Can you work these out from the model? Positions are in its coordinate system, mm. A direction names the side the tool comes from. Give positions to 0.01 mm unless a question says otherwise; leave off trailing zeros. Write each loop counter-clockwise with the first axis right and the second up, starting at its lowest first coordinate (ties: lowest second). Pieces come first, ordered by that corner, then holes.
from build123d import *

# Parameters (mm, degrees)
F0_W     = 304.8
F0_H     = 6.35
F1_DEPTH = 50.8
F3_DEPTH = 0.8125
F5_DEPTH = 20.6502


# Not quite as in the source:
# - a pattern or mirror of a feature is missing from the dataset's text; its kind, count and spacing are read off the source's solid


with BuildPart() as f1:
    # F0 (on Right) → F1 (new body)
    with BuildSketch(Plane.YZ):
        with BuildLine():
            Line((-304.8, 6.35), (0, 6.35))
            Line((0, 6.35), (0, 19.05))
            ThreePointArc((0, 19.05), (-152.4, 44.45), (-304.8, 19.05))
            Line((-304.8, 19.05), (-304.8, 6.35))
        make_face()
        with BuildLine():
            ThreePointArc((-304.8, 19.05), (-152.4, 44.45), (0, 19.05))
            Line((0, 19.05), (0, 25.4))
            ThreePointArc((0, 25.4), (-152.4, 50.8), (-304.8, 25.4))
            Line((-304.8, 25.4), (-304.8, 19.05))
        make_face()
        with Locations((-152.4, 3.175)):
            Rectangle(F0_W, F0_H)
    extrude(amount=F1_DEPTH)

    # F2 (on face) → F3 (cut)
    with BuildSketch(Plane.YZ.offset(50.8)):
        with BuildLine():
            Line((0, 6.35), (0, 19.05))
            ThreePointArc((0, 19.05), (-152.4, 44.45), (-304.8, 19.05))
            Line((-304.8, 19.05), (-304.8, 6.35))
            Line((-304.8, 6.35), (0, 6.35))
        make_face()
    extrude(amount=-F3_DEPTH, mode=Mode.SUBTRACT)

    # F4 (on face) → F5 (cut)
    with BuildSketch(Plane(origin=(0, 0, 0), x_dir=(0, -1, 0), z_dir=(-1, 0, 0))):
        with BuildLine():
            Line((304.8, 6.35), (304.8, 19.05))
            ThreePointArc((304.8, 19.05), (152.4, 44.45), (0, 19.05))
            Line((0, 19.05), (0, 6.35))
            Line((0, 6.35), (304.8, 6.35))
        make_face()
    f5 = extrude(amount=-F5_DEPTH, mode=Mode.SUBTRACT)

    # F5_copies: F5 across plane
    add(f5.mirror(Plane(origin=(25.40635, 0, 0), x_dir=(0, 0, 1), z_dir=(1, 0, 0))), mode=Mode.SUBTRACT)


solid = f1.part
(1) Imagine slicing it at B-B, the plane y = -109. Write out the boundary of the cut face in (x, z), plus the area to 3 significant figures.
Returned:
outline: (0, 0) - (50.8, 0) - (50.8, 6.35) - (30.16, 6.35) - (30.16, 42.44) - (50.8, 42.44) - (50.8, 48.79) - (0, 48.79) - (0, 42.44) - (20.65, 42.44) - (20.65, 6.35) - (0, 6.35) - close
area: 988 mm2
(2) For faces 1 (the face through (50.8, -153, 47)), 2 (the face through (10.181, -154.573, 44.445)), 3 (the face through (41, -150, 6.35)), 4 (the face through (10, -150, 6.35)), which set-ups out of +Z, -Z, +X, -X, +Y, -Y let a thin tool reach every point of the face, with its end or its side?
Returned:
face 1: +Z, -Z, +X, +Y, -Y
face 2: -X
face 3: +X, +Y, -Y
face 4: -X, +Y, -Y
(3) If I drill on L1, parallel to Z at x = 9.5, y = -151.5; L2, parallel to Z at x = 31.5, y = -268.5; L3, parallel to X at y = -92, z = 20.5, over which ranges is the centre line in solid material (lowest first)?
Returned:
L1: z = 0 to 6.35, 44.45 to 50.8
L2: z = 0 to 6.35, 29.88 to 36.23
L3: x = 20.65 to 30.16
(4) If we mould it in two halves opening along Y, with no side actions, what happens to faces 5 (the face through (25.044, -150.227, 50.795)), 6 (the face through (25, -155, 0)), 7 (the face through (30.162, -150, 21)), 8 (the face through (40.626, -150.227, 44.445))? For each: +Y half, -Y half, draft (parallel to the pull), parting line (faces both ways), or undercut.
Returned:
face 5: parting line
face 6: draft
face 7: undercut
face 8: undercut
(5) Imagine slicing it at C-C, the plane z = 31. Write out the boundary of the cut face in (x, y), plus the area to 3 significant figures.
Returned:
outline: (0, -287.37) - (50.8, -287.37) - (50.8, -264.02) - (30.16, -264.02) - (30.16, -40.78) - (50.8, -40.78) - (50.8, -17.43) - (0, -17.43) - (0, -40.78) - (20.65, -40.78) - (20.65, -264.02) - (0, -264.02) - close
area: 4,500 mm2
(6) Imagine slicing it at A-A, the plane x = 40. Write out the boundary of the cut face in (y, z).
Returned:
outline: (-304.8, 0) - (0, 0) - (0, 6.35) - (-304.8, 6.35) - close; (-304.8, 19.05) arc R469.9 cw to (0, 19.05) - (0, 25.4) arc R469.9 ccw to (-304.8, 25.4) - close
(7) Will these pins go through, and if not, where does the flat tip stop? P1, Ø10, axis at y = -110.5, z = 16, coming from the -X side; P2, Ø11.5, axis at y = -83, z = 25, coming from the +X side.
Returned:
P1: stops at x = 20.65
P2: stops at x = 30.16
